```python
from build123d import *

# Parameters (mm, degrees)
BOSS_EXTRUDE1_DEPTH = 62.992
CUT_EXTRUDE1_DEPTH  = 57.912
BOSS_EXTRUDE2_DEPTH = 40.132
CUT_EXTRUDE2_DEPTH  = 40.132
CUT_EXTRUDE3_DEPTH  = 35.052
BOSS_EXTRUDE3_DEPTH = 2.54
CUT_EXTRUDE4_DEPTH  = 2.54
CHAMFER1_SIZE       = 4.92
CHAMFER3_SIZE       = 2.38
CHAMFER4_SIZE       = 2.38
SKETCH12_R          = 2
CUT_EXTRUDE6_DEPTH  = 2.54
SKETCH16_R          = 2.032
CUT_EXTRUDE7_DEPTH  = 2.54


with BuildPart() as part:
    # Sketch2 → Boss-Extrude1 (new body)
    with BuildSketch(Plane.XY):
        with BuildLine():
            Line((-23.622, 0), (23.622, 0))
            ThreePointArc((23.622, 0), (0, -23.622), (-23.622, 0))
        make_face()
    extrude(amount=-BOSS_EXTRUDE1_DEPTH)

    # Sketch3 → Cut-Extrude1 (cut)
    with BuildSketch(Plane.XY):
        with BuildLine():
            Line((-18.542, 0), (18.542, 0))
            ThreePointArc((18.542, 0), (0, -18.542), (-18.542, 0))
        make_face()
    extrude(amount=-CUT_EXTRUDE1_DEPTH, mode=Mode.SUBTRACT)

    # Sketch5 → Boss-Extrude2 (add)
    with BuildSketch(Plane.XY):
        with BuildLine():
            Line((-33.782, 0), (33.782, 0))
            ThreePointArc((33.782, 0), (0, -33.782), (-33.782, 0))
        make_face()
    extrude(amount=BOSS_EXTRUDE2_DEPTH)

    # Sketch6 → Cut-Extrude2 (cut)
    with BuildSketch(Plane.XY.offset(40.132)):
        with BuildLine():
            Line((-18.542, 0), (18.542, 0))
            ThreePointArc((18.542, 0), (0, -18.542), (-18.542, 0))
        make_face()
    extrude(amount=-CUT_EXTRUDE2_DEPTH, mode=Mode.SUBTRACT)

    # Sketch7 → Cut-Extrude3 (cut)
    with BuildSketch(Plane.XY.offset(40.132)):
        with BuildLine():
            Line((-28.702, 0), (28.702, 0))
            ThreePointArc((28.702, 0), (0, -28.702), (-28.702, 0))
        make_face()
    extrude(amount=-CUT_EXTRUDE3_DEPTH, mode=Mode.SUBTRACT)

    # Sketch9 → Boss-Extrude3 (add)
    with BuildSketch(Plane.XY.offset(40.132)):
        with BuildLine():
            Line((-41.402, 0), (41.402, 0))
            ThreePointArc((41.402, 0), (0, -41.402), (-41.402, 0))
        make_face()
    extrude(amount=-BOSS_EXTRUDE3_DEPTH)

    # Sketch10 → Cut-Extrude4 (cut)
    with BuildSketch(Plane.XY.offset(40.132)):
        with BuildLine():
            Line((-28.702, 0), (28.702, 0))
            ThreePointArc((28.702, 0), (0, -28.702), (-28.702, 0))
        make_face()
    extrude(amount=-CUT_EXTRUDE4_DEPTH, mode=Mode.SUBTRACT)

    # Chamfer1
    chamfer1_edges = [part.edges().sort_by_distance(p)[0] for p in [
        (0, -23.622, 0),
    ]]
    chamfer(chamfer1_edges, length=CHAMFER1_SIZE)

    # Chamfer3
    chamfer3_edges = [part.edges().sort_by_distance(p)[0] for p in [
        (0, -23.622, -62.992),
    ]]
    chamfer(chamfer3_edges, length=CHAMFER3_SIZE)

    # Chamfer4
    chamfer4_edges = [part.edges().sort_by_distance(p)[0] for p in [
        (0, -33.782, 0),
    ]]
    chamfer(chamfer4_edges, length=CHAMFER4_SIZE)

    # Sketch12 → Cut-Extrude6 (cut)
    with BuildSketch(Plane(origin=(0, 0, 37.592), x_dir=(-1, 0, 0), z_dir=(0, 0, -1))):
        with Locations((0, -37.592)):
            Circle(SKETCH12_R)
    extrude(amount=-CUT_EXTRUDE6_DEPTH, mode=Mode.SUBTRACT)

    # Sketch16 → Cut-Extrude7 (cut)
    with BuildSketch(Plane.XY.offset(40.132)):
        with Locations((-33.156425447, -17.714680792)):
            Circle(SKETCH16_R)
        with Locations((33.359405316, -17.329412596)):
            Circle(SKETCH16_R)
    extrude(amount=-CUT_EXTRUDE7_DEPTH, mode=Mode.SUBTRACT)


solid = part.part
```
Here's how the part is built. I have some questions about the finished solid (model axes, mm). A direction names the side the tool comes from. Give positions to 0.01 mm unless a question says otherwise; leave off trailing zeros. Order: outer loops, then holes, each group sorted by start corner. A loop starts at its lowest first (then second) coordinate and runs counter-clockwise, first axis right, second up. Notation, with made-up numbers: (32, -35.75) - (86, -35.75) arc R19 ccw to (86, -21.75) - close; hole circle Ø5 at (-11.75, 21). An arc over 180 degrees is marked (long way). Answer as a JSON object with one key per item and string values. Group by question number.
Item 1: If we section it at C-C on z = -7.5: Please give me the cut outline in (x, y), and give its area (3 significant figures).
Item 2: If we section it at B-B on z = 23: Please give me the cut outline in (x, y), and give its area (3 significant figures).
Item 3: If we section it at A-A on x = 0: Please give me the cut outline in (y, z), and give its area (3 significant figures).
Item 4: If we mould it in two halves opening along X, with no side actions, what happens to faces 4 (the flat face through (-19, 0, -11)), 5 (the cylindrical face through (0.743, -33.774, 19.74)), 6 (the flat face through (0, -7, -57.912))? For each: pulls with the +X half, pulls with the -X half, needs draft (parallel to the pull), parting line crosses it, or undercut.
Item 5: For P1, Ø1.5, axis at y = -23.5, z = 27, coming from the +X side; P2, Ø1, axis at y = -29.5, z = 16.5, coming from the +X side; P3, Ø5, axis at x = 1, y = -28, coming from the -Z side, each with a flat end and sliding along its axis, tell me the tip position at first contact or that it passes through.
Item 6: Please list where these lines run through material, in increasing order: probe 1 along Z at (x, y) = (7, -13.5); probe 2 along Z at (x, y) = (2.5, -38); probe 3 along X at (y, z) = (-15, -57).
Item 7: Which directions (+Z, -Z, +X, -X, +Y, -Y) give clear straight access to the entire face, cutting with the end or side of a thin tool? Please do faces 1 (the flat face through (0, -21, 5.08)), 2 (the cylindrical face through (0.91, -41.39, 38.88)), 3 (the cylindrical face through (0.519, -23.616, -32.376)).
Result set:
{
 "1": {"outline": "(-23.62, 0) arc R23.62 ccw to (23.62, 0) - (18.54, 0) arc R18.54 cw to (-18.54, 0) - close", "area": "336 mm²"},
 "2": {"outline": "(-33.78, 0) arc R33.78 ccw to (33.78, 0) - (28.7, 0) arc R28.7 cw to (-28.7, 0) - close", "area": "499 mm²"},
 "3": {"outline": "(-41.4, 37.59) - (-39.59, 37.59) - (-39.59, 40.13) - (-41.4, 40.13) - close; (-35.59, 37.59) - (-33.78, 37.59) - (-33.78, 2.38) - (-31.4, 0) - (-28.54, 0) - (-23.62, -4.92) - (-23.62, -60.61) - (-21.24, -62.99) - (0, -62.99) - (0, -57.91) - (-18.54, -57.91) - (-18.54, 5.08) - (-28.7, 5.08) - (-28.7, 40.13) - (-35.59, 40.13) - close", "area": "685 mm²"},
 "4": {"face 4": "needs draft", "face 5": "parting line crosses it", "face 6": "undercut"},
 "5": {"P1": "x = 24.97", "P2": "x = 17.33", "P3": "z = -3.02"},
 "6": {"probe 1": "-62.99 to -57.91", "probe 2": "37.59 to 40.13", "probe 3": "-18.25 to -10.9, 10.9 to 18.25"},
 "7": {"face 1": "+Z, +Y", "face 2": "+Z, -Z, -Y", "face 3": "-Z, -Y"}
}
